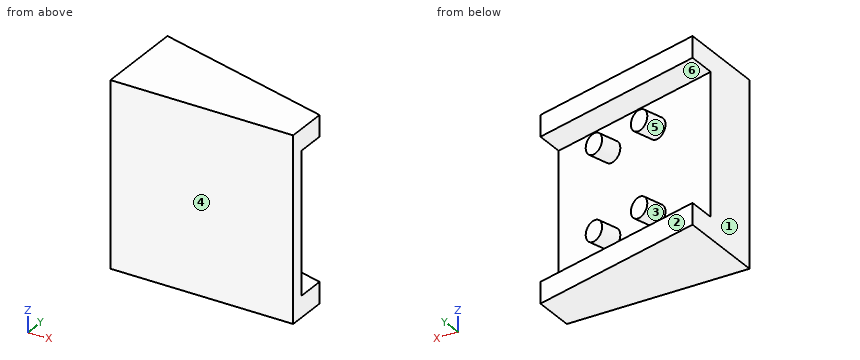
from build123d import *

# Parameters (mm, degrees)
SKETCH1_W           = 26
SKETCH1_H           = 26
BOSS_EXTRUDE1_DEPTH = 12.966679003
CUT_EXTRUDE1_DEPTH  = 39.988905658
SKETCH3_W           = 50
SKETCH3_H           = 20
CUT_EXTRUDE2_DEPTH  = 4
SKETCH5_R           = 1.45
BOSS_EXTRUDE2_DEPTH = 3


with BuildPart() as part:
    # Sketch1 → Boss-Extrude1 (new body)
    with BuildSketch(Plane(origin=(0, 0, 0), x_dir=(1, 0, 0), z_dir=(0, 1, 0))):
        with Locations((13, 13)):
            Rectangle(SKETCH1_W, SKETCH1_H)
    extrude(amount=BOSS_EXTRUDE1_DEPTH)

    # Sketch2 → Cut-Extrude1 (cut, through all)
    with BuildSketch(Plane.XY):
        Polygon((0, 12.966679003), (26, 6), (26, 12.966679003), align=None)
    extrude(amount=-CUT_EXTRUDE1_DEPTH, mode=Mode.SUBTRACT)

    # Sketch3 → Cut-Extrude2 (cut)
    with BuildSketch(Plane(origin=(3.241669751, 12.098076211, 0), x_dir=(0.9659258262890681, -0.25881904510252174, 0), z_dir=(0.2588190451025217, 0.965925826289068, 0))):
        with Locations((21.643976522, 13)):
            Rectangle(SKETCH3_W, SKETCH3_H)
    extrude(amount=-CUT_EXTRUDE2_DEPTH, mode=Mode.SUBTRACT)

    # Sketch5 → Boss-Extrude2 (add)
    with BuildSketch(Plane(origin=(2.20639357, 8.234372906, 0), x_dir=(0.9659258262890681, -0.2588190451025218, 0), z_dir=(0.25881904510252174, 0.965925826289068, 0))):
        with Locations((7.174363637, 19)):
            Circle(SKETCH5_R)
        with Locations((7.174363637, 7)):
            Circle(SKETCH5_R)
        with Locations((15.174363637, 19)):
            Circle(SKETCH5_R)
        with Locations((15.174363637, 7)):
            Circle(SKETCH5_R)
    extrude(amount=BOSS_EXTRUDE2_DEPTH)


solid = part.part
Source: CAD feature listing. Evaluate the final solid. Frame: model axes, mm. Face numbers are marked on the shaded views. A direction names the side the tool comes from. Coordinates: 2 decimals unless noted, no trailing zeros. Loops run counter-clockwise (first coordinate to the right, second up) from the corner with the lowest first, then second, coordinate; pieces in that order, holes last. Notation, with made-up numbers: (-13, 1.25) -> (2, 1.25) arc R24 cw to (2, 37.25) -> close; hole circle Ø5 at (21.5, 70). An arc over 180 degrees is marked (long way). Answer in a Markdown table with one row per item. Add a question column.
Q1. Contact query for flat-ended pins moving along their axis: pin 1 Ø1 at (x, z) = (6, -9) entering from +Y; pin 2 Ø1.5 at (x, z) = (13.5, -8) entering from +Y. Output: stop coordinate, or through.
Q2. Section C-C on z = -4. Return the cut outline in (x, y).
Q3. Section D-D on y = 3. Return the cut outline in (x, z).
Q4. Reachability of the marked faces 5 and 6 from +Z, -Z, +X, -X, +Y, -Y: full face, straight path, thin tool, end or side. Return the list, or none.
Q5. Pull-direction query (Y, two-part tool) for the marked faces 1, 2, 3 and 4; classes: pulls with the +Y half, pulls with the -Y half, needs draft (parallel to the pull), parting line crosses it, or undercut.
Q6. Section A-A on y = 11.5. Return the cut outline in (x, z), and give its area (3 significant figures).
Q7. Section B-B on x = 21.75. Return the cut outline in (y, z).
Q8. Ray query, line 1 along Z through (x, y) = (3.25, 8.5); line 2 along Y through (x, z) = (13.25, -21); line 3 along Y through (x, z) = (25, -18.5). Return the intervals inside material, ascending.
Computed values:
| question | item | result |
|---|---|---|
| 1 | pin 1 | stops at y = 7.35 |
| 1 | pin 2 | stops at y = 5.41 |
| 2 | outline | (0, 0) -> (26, 0) -> (26, 1.86) -> (0, 8.83) -> close |
| 3 | outline | (0, -26) -> (26, -26) -> (26, -23) -> (21.74, -23) -> (21.74, -3) -> (26, -3) -> (26, 0) -> (0, 0) -> close |
| 4 | face 5 | none |
| 4 | face 6 | +X, +Y |
| 5 | face 1 | needs draft |
| 5 | face 2 | pulls with the +Y half |
| 5 | face 3 | undercut |
| 5 | face 4 | pulls with the -Y half |
| 6 | outline | (0, -26) -> (5.47, -26) -> (5.47, -23) -> (0, -23) -> close; (0, -3) -> (5.47, -3) -> (5.47, 0) -> (0, 0) -> close |
| 6 | area | 32.8 mm^2 |
| 7 | outline | (0, -26) -> (7.14, -26) -> (7.14, -23) -> (3, -23) -> (3, -3) -> (7.14, -3) -> (7.14, 0) -> (0, 0) -> close |
| 8 | line 1 | z = -26 to -23, -3 to 0 |
| 8 | line 2 | y = 0 to 5.28 |
| 8 | line 3 | y = 0 to 2.13 |
